Geometry check sheet. Reference: the model listing, model coordinates, mm. Coordinates: 2 decimals unless noted, no trailing zeros. Order: outer loops, then holes, each group sorted by start corner. A loop starts at its lowest first (then second) coordinate and runs counter-clockwise, first axis right, second up. Notation, with made-up numbers: (25, 19.5) - (65, 19.5) arc R24 cw to (65, 58.5) - close; hole circle Ø4 at (74, 19.5). An arc over 180 degrees is marked (long way). Use CSV: the item, a comma, the result in double quotes. Start each with the question number.
1) Thickness scan on probe 1 along Z at (x, y) = (-8.5, -15.5); probe 2 along Y at (x, z) = (-27, 17); probe 3 along X at (y, z) = (-30, 33). Record the ranges inside material, lowest first. Write a range as [from, to].
2) Draft check along Y on faces 1 (the conical face through (68.24, -43.5, 81.24)), 2 (the flat face through (-57, 63, 161.716)), 3 (the flat face through (1, -1, 5.123)). Enter one of: released by +Y, released by -Y, zero draft, split by the parting line, or undercut.
3) Sectioned sample at A-A, the plane x = 0. Record the cut outline in (y, z) (3 decimals), and give its area (3 significant figures).
4) Sectioned sample at C-C, the plane z = 69.5. Record the cut outline in (x, y), and give its area (3 significant figures).
5) Sectioned sample at D-D, the plane z = 126.5. Record the cut outline in (x, y).
6) Depth check by flat-ended pin: P1, Ø8, axis at x = -49.5, z = 125, coming from the +Y side; P2, Ø1, axis at x = 22.5, y = -3.5, coming from the +Z side; P3, Ø2, axis at y = 29.5, z = 55, coming from the -X side. Enter the tip coordinate at first touch or a pass-through.
from build123d import *


with BuildPart() as f1:
    # F0 (on Right) → F1 (revolve)
    with BuildSketch(Plane.YZ):
        with BuildLine():
            Line((-73.025, 0), (0, 0))
            Line((0, 0), (0, 5.122894))
            Line((0, 5.122894), (-66.973096, 5.122894))
            ThreePointArc((-66.973096, 5.122894), (-69.149371, 5.986086), (-70.142311, 8.106309))
            Line((-70.142311, 8.106309), (-79.13973, 156.942341))
            ThreePointArc((-79.13973, 156.942341), (-80.728433, 160.334697), (-84.210473, 161.715805))
            Line((-84.210473, 161.715805), (-85.789887, 161.715805))
            Line((-85.789887, 161.715805), (-76.194214, 2.983415))
            ThreePointArc((-76.194214, 2.983415), (-75.201275, 0.863193), (-73.025, 0))
        make_face()
    revolve(axis=Axis((0, 0, 2.561447), (0, 0, 1)))


solid = f1.part
Evaluation:
1,probe 1,"[0, 5.12]"
1,probe 2,"[-72.16, -65.32], [65.32, 72.16]"
1,probe 3,"[-72.01, -65.06], [65.06, 72.01]"
2,face 1,"split by the parting line"
2,face 2,"zero draft"
2,face 3,"undercut"
3,outline,"(-85.79, 161.716) - (-76.194, 2.983) arc R3.175 ccw to (-73.025, 0) - (73.025, 0) arc R3.175 ccw to (76.194, 2.983) - (85.79, 161.716) - (84.21, 161.716) arc R5.08 ccw to (79.14, 156.942) - (70.142, 8.106) arc R3.175 cw to (66.973, 5.123) - (-66.973, 5.123) arc R3.175 cw to (-70.142, 8.106) - (-79.14, 156.942) arc R5.08 ccw to (-84.21, 161.716) - close"
3,area,"2,760 mm²"
4,outline,"circle Ø160.43 at (0, 0); hole circle Ø147.71 at (0, 0)"
4,area,"3,080 mm²"
5,outline,"circle Ø167.32 at (0, 0); hole circle Ø154.6 at (0, 0)"
6,P1,"y = 70.11"
6,P2,"z = 5.12"
6,P3,"x = -74.05"
